The model under review builds one solid part; all positions refer to its coordinate system, in mm. A direction names the side the tool comes from. Give positions to 0.01 mm unless a question says otherwise; leave off trailing zeros. Loops run counter-clockwise (first coordinate to the right, second up) from the corner with the lowest first, then second, coordinate; pieces in that order, holes last. Notation, with made-up numbers: M 71,86.5 L 99,86.5 A20 cw 99,113.5 Z; hole C -36.5,78.25 d3. An arc over 180 degrees is marked long. Write item = value, one per line. Start each with the question number.
1. We need section A-A on y = -6. Give the boundary of the cut face in (x, z).
2. Wall thickness on line 1 along Z through (x, y) = (-0.75, 9.25); line 2 along Y through (x, z) = (0.25, 24); line 3 along X through (y, z) = (1.5, 32): over which ranges is each line inside the solid? List them lowest first. Write a range as from..to.
3. Draft analysis for pull direction Z (two halves, no side actions). For faces 3 (the face through (0, 0, 55)), 4 (the face through (-1.08, -4.88, 24.65)), 5 (the face through (-5, -2, 50)), 6 (the face through (2.17, -9.76, -2.46)), state which applies: pulls with the +Z half, pulls with the -Z half, needs draft (parallel to the pull), parting line crosses it, or undercut.
4. We need section D-D on x = 6.5. Give the boundary of the cut face in (y, z).
5. For faces 1 (the face through (5, -2, 0)), 2 (the face through (0, 0, -5)), list the 3-axis set-ups (+Z, -Z, +X, -X, +Y, -Y) from which the entire face can be reached by the end or side of a thin tool; tool diameter is ignored.
6. We need section B-B on x = 0. Give the boundary of the cut face in (y, z), then the cut area to 3 significant figures.
7. For pin 1 (1 mm diameter, centred on y = -5, z = 46.5, fed in from +X); pin 2 (6 mm diameter, centred on y = -4.5, z = 26.5, fed in from -X); pin 3 (5 mm diameter, centred on y = -5, z = 1.5, fed in from +X), all flat-tipped, find the tip position at first contact; note any pin that passes through.
from build123d import *

# Parameters (mm, degrees)
SKETCH2_R           = 5
BOSS_EXTRUDE1_DEPTH = 50
SKETCH3_R           = 10
BOSS_EXTRUDE2_DEPTH = 5
SKETCH4_R           = 10
BOSS_EXTRUDE3_DEPTH = 5


with BuildPart() as part:
    # Sketch2 → Boss-Extrude1 (new body)
    with BuildSketch(Plane.XY):
        Circle(SKETCH2_R)
    extrude(amount=BOSS_EXTRUDE1_DEPTH)

    # Sketch3 → Boss-Extrude2 (add)
    with BuildSketch(Plane(origin=(0, 0, 0), x_dir=(-1, 0, 0), z_dir=(0, 0, -1))):
        Circle(SKETCH3_R)
    extrude(amount=BOSS_EXTRUDE2_DEPTH)

    # Sketch4 → Boss-Extrude3 (add)
    with BuildSketch(Plane.XY.offset(50)):
        Circle(SKETCH4_R)
    extrude(amount=BOSS_EXTRUDE3_DEPTH)


solid = part.part
Final values:
q1.outline = M -8,-5 L 8,-5 L 8,0 L -8,0 Z; M -8,50 L 8,50 L 8,55 L -8,55 Z
q2.line_1 = -5..0, 50..55
q2.line_2 = -4.99..4.99
q2.line_3 = -4.77..4.77
q3.face_3 = pulls with the +Z half
q3.face_4 = undercut
q3.face_5 = undercut
q3.face_6 = needs draft
q4.outline = M -7.6,-5 L 7.6,-5 L 7.6,0 L -7.6,0 Z; M -7.6,50 L 7.6,50 L 7.6,55 L -7.6,55 Z
q5.face_1 = none
q5.face_2 = -Z, +X, -X, +Y, -Y
q6.outline = M -10,-5 L 10,-5 L 10,0 L 5,0 L 5,50 L 10,50 L 10,55 L -10,55 L -10,50 L -5,50 L -5,0 L -10,0 Z
q6.area = 700 mm²
q7.pin_1 = 2.18
q7.pin_2 = -4.77
q7.pin_3 = 9.54
